```python
from build123d import *

# Parameters (mm, degrees)
BOSS_EXTRUDE1_DEPTH = 285.75
SKETCH2_R           = 1.27
CUT_EXTRUDE1_DEPTH  = 20.05
SKETCH4_R           = 3.175
CUT_EXTRUDE2_DEPTH  = 140.208
SKETCH5_R           = 6.35
CUT_EXTRUDE3_DEPTH  = 2.54


with BuildPart() as part:
    # Sketch1 → Boss-Extrude1 (new body, symmetric)
    with BuildSketch(Plane(origin=(0, 0, 0), x_dir=(1, 0, 0), z_dir=(0, 1, 0))):
        Polygon((19.05, 3.81), (19.05, 6.35), (0, 6.35), (0, -6.35), (19.05, -6.35), (19.05, -3.81), (2.54, -3.81), (2.54, 3.81), align=None)
    extrude(amount=BOSS_EXTRUDE1_DEPTH, both=True)

    # Sketch2 → Cut-Extrude1 (cut, through all)
    with BuildSketch(Plane.ZY):
        with Locations((-0.286445318, 279.4)):
            Circle(SKETCH2_R)
        with Locations((-0.286445318, 222.25)):
            Circle(SKETCH2_R)
        with Locations((-0.286445318, 165.1)):
            Circle(SKETCH2_R)
        with Locations((-0.286445318, 107.95)):
            Circle(SKETCH2_R)
        with Locations((-0.286445318, 50.8)):
            Circle(SKETCH2_R)
        with Locations((-0.286445318, -6.35)):
            Circle(SKETCH2_R)
        with Locations((-0.286445318, -63.5)):
            Circle(SKETCH2_R)
        with Locations((-0.286445318, -120.65)):
            Circle(SKETCH2_R)
        with Locations((-0.286445318, -177.8)):
            Circle(SKETCH2_R)
        with Locations((-0.286445318, -234.95)):
            Circle(SKETCH2_R)
    extrude(amount=-CUT_EXTRUDE1_DEPTH, mode=Mode.SUBTRACT)

    # Sketch4 → Cut-Extrude2 (cut)
    with BuildSketch(Plane(origin=(0, 0, 3.81), x_dir=(-1, 0, 0), z_dir=(0, 0, -1))):
        with Locations((-9.525, 260.35)):
            Circle(SKETCH4_R)
        with Locations((-9.525, 86.868)):
            Circle(SKETCH4_R)
        with Locations((-9.525, -86.614)):
            Circle(SKETCH4_R)
        with Locations((-9.525, -260.096)):
            Circle(SKETCH4_R)
    extrude(amount=-CUT_EXTRUDE2_DEPTH, mode=Mode.SUBTRACT)

    # Sketch5 → Cut-Extrude3 (cut)
    with BuildSketch(Plane(origin=(0, 0, -6.35), x_dir=(-1, 0, 0), z_dir=(0, 0, -1))):
        with Locations((-9.525, 260.35)):
            Circle(SKETCH5_R)
        with Locations((-9.525, 86.7918)):
            Circle(SKETCH5_R)
        with Locations((-9.525, -86.7664)):
            Circle(SKETCH5_R)
        with Locations((-9.525, -260.3246)):
            Circle(SKETCH5_R)
    extrude(amount=-CUT_EXTRUDE3_DEPTH, mode=Mode.SUBTRACT)


solid = part.part
```
The model under review builds one solid part; all positions refer to its coordinate system, in mm. A direction names the side the tool comes from. Coordinates: 2 decimals unless noted, no trailing zeros. Write each loop counter-clockwise with the first axis right and the second up, starting at its lowest first coordinate (ties: lowest second). Pieces come first, ordered by that corner, then holes. Notation, with made-up numbers: (-32.5, 56) - (-25.5, 56) arc R10 cw to (-25.5, 63) - close; hole circle Ø10 at (31.25, 84.5). An arc over 180 degrees is marked (long way). Answer in a Markdown table with one row per item. Add a question column.
Q1. To check wall thickness, follow line 1 along Z through (x, y) = (3.25, -46); line 2 along Y through (x, z) = (12.25, -4); line 3 along Z through (x, y) = (0.8, -120.65). State the ranges of each line that lie inside material, in increasing order. Write a range as from..to.
Q2. Clearance check with flat-ended pins moving along their axes: pin 1 (4 mm diameter, centred on y = 279.4, z = -0.29, fed in from -X); pin 2 (2 mm diameter, centred on y = -6.35, z = -0.29, fed in from +X); pin 3 (7.5 mm diameter, centred on x = 9.525, y = 260.35, fed in from -Z); pin 4 (2.5 mm diameter, centred on y = -89, z = 1.5, fed in from +X). State where each tip first meets the part, or that it passes through.
Q3. Consider section A-A on y = 4.5. Give the boundary of the cut face in (x, z).
Q4. For faces 1 (the face through (10.902, 80.593, -5.098)), 2 (the face through (11, 4, 3.81)), 3 (the face through (0, 4, 0)), list the 3-axis set-ups (+Z, -Z, +X, -X, +Y, -Y) from which the entire face can be reached by the end or side of a thin tool; tool diameter is ignored.
Q5. Draft analysis for pull direction Y (two halves, no side actions). For faces 4 (the face through (10.352, 266.646, -5.098)), 5 (the face through (9, 4, 6.35)), 6 (the face through (10.902, -266.524, -5.098)), 7 (the face through (9, 285.75, -4)), state which applies: +Y half, -Y half, draft (parallel to the pull), parting line (faces both ways), or undercut.
Q6. Consider section B-B on x = 9.5. Give the number of separate pieces and of enclosed holes in the cut face, then the cut area to 3 significant figures.
Answers below:
| question | item | result |
|---|---|---|
| 1 | line 1 | -6.35..-3.81, 3.81..6.35 |
| 1 | line 2 | -285.75..-266.06, -254.59..-92.5, -81.03..81.06, 92.53..254.61, 266.09..285.75 |
| 1 | line 3 | -6.35..-1.56, 0.98..6.35 |
| 2 | pin 1 | x = 0 |
| 2 | pin 2 | through |
| 2 | pin 3 | z = 3.81 |
| 2 | pin 4 | x = 2.54 |
| 3 | outline | (0, -6.35) - (19.05, -6.35) - (19.05, -3.81) - (2.54, -3.81) - (2.54, 3.81) - (19.05, 3.81) - (19.05, 6.35) - (0, 6.35) - close |
| 4 | face 1 | -Z |
| 4 | face 2 | +X, +Y, -Y |
| 4 | face 3 | +Z, -Z, -X, +Y, -Y |
| 5 | face 4 | undercut |
| 5 | face 5 | draft |
| 5 | face 6 | undercut |
| 5 | face 7 | +Y half |
| 6 | separate pieces | 10 |
| 6 | enclosed holes | 0 |
| 6 | area | 2,710 mm² |
